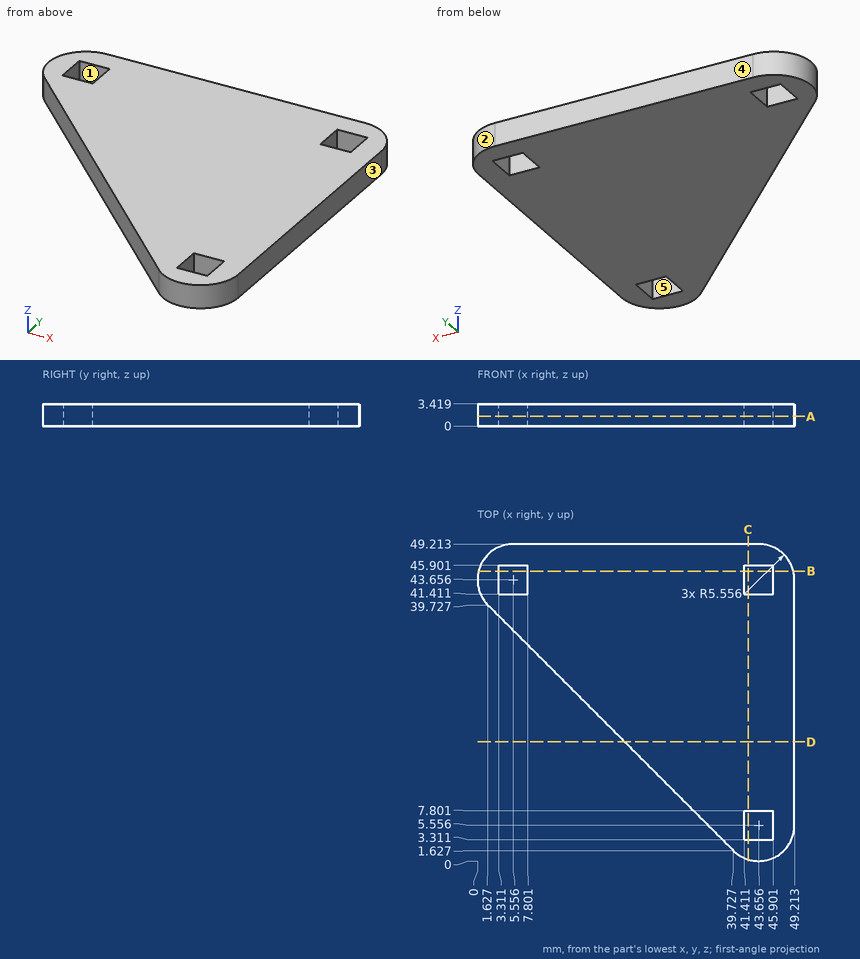
Source: three-view drawing plus pictorial views. Frame: mm from the lowest corner of the part. A direction names the side the tool comes from. Round coordinates to 2 decimals unless told otherwise and drop trailing zeros. Order: outer loops, then holes, each group sorted by start corner. A loop starts at its lowest first (then second) coordinate and runs counter-clockwise, first axis right, second up. Notation, with made-up numbers: (37.5, 24) -> (81.5, 24) arc R20 ccw to (81.5, 46) -> close; hole circle Ø9 at (67, 70). An arc over 180 degrees is marked (long way). Use CSV: the item, a comma, the result in double quotes. Start each with the question number.
1) Material intervals for line 1 along X through (y, z) = (44, 2.8); line 2 along X through (y, z) = (41.5, 2.4) (1 decimal), sorted ascending. Write a range as from..to.
2) Section D-D (y = 18.5). Return the cut outline in (x, z) (1 decimal).
3) Draft query along Y for the marked faces 1, 2 and 3. Return one class per face: +Y half, -Y half, draft (parallel to the pull), parting line (faces both ways), or undercut.
4) Section B-B (y = 45). Return the cut outline in (x, z) (1 decimal).
5) Set-up query: the marked faces 4 and 5. Return all of +Z, -Z, +X, -X, +Y, -Y with unobstructed straight access to the full face (end or side cutting, diameter ignored); none if empty.
6) Section C-C (x = 42). Return the cut outline in (y, z), and give its area (3 significant figures).
7) First-contact query: pin 1 Ø1.7 at (y, z) = (43, 1.5) entering from -X; pin 2 Ø1.5 at (x, z) = (12.5, 2.5) entering from -Y (1 decimal); pin 3 Ø1 at (y, z) = (4.5, 1.5) entering from -X (1 decimal). Flat tips, straight axial feed; report the tip coordinate or a pass-through.
8) Section A-A (z = 1.5). Return the cut outline in (x, y).
Returned:
1,line 1,"x = 0.01..3.31, 7.8..41.41, 45.9..49.2"
1,line 2,"x = 0.4..3.3, 7.8..41.4, 45.9..49.2"
2,outline,"(22.9, 0) -> (49.2, 0) -> (49.2, 3.4) -> (22.9, 3.4) -> close"
3,face 1,"undercut"
3,face 2,"+Y half"
3,face 3,"draft"
4,outline,"(0.2, 0) -> (3.3, 0) -> (3.3, 3.4) -> (0.2, 3.4) -> close; (7.8, 0) -> (41.4, 0) -> (41.4, 3.4) -> (7.8, 3.4) -> close; (45.9, 0) -> (49, 0) -> (49, 3.4) -> (45.9, 3.4) -> close"
5,face 4,"+Z, -Z, +X, -X, +Y"
5,face 5,"+Z, -Z"
6,outline,"(0.25, 0) -> (3.31, 0) -> (3.31, 3.42) -> (0.25, 3.42) -> close; (7.8, 0) -> (41.41, 0) -> (41.41, 3.42) -> (7.8, 3.42) -> close; (45.9, 0) -> (49.21, 0) -> (49.21, 3.42) -> (45.9, 3.42) -> close"
6,area,"137 mm²"
7,pin 1,"stops at x = 0"
7,pin 2,"stops at y = 28.1"
7,pin 3,"stops at x = 36.4"
8,outline,"(1.63, 39.73) -> (39.73, 1.63) arc R5.56 ccw to (49.21, 5.56) -> (49.21, 43.66) arc R5.56 ccw to (43.66, 49.21) -> (5.56, 49.21) arc R5.56 ccw to start; hole (3.31, 41.41) -> (7.8, 41.41) -> (7.8, 45.9) -> (3.31, 45.9) -> close; hole (41.41, 3.31) -> (45.9, 3.31) -> (45.9, 7.8) -> (41.41, 7.8) -> close; hole (41.41, 41.41) -> (45.9, 41.41) -> (45.9, 45.9) -> (41.41, 45.9) -> close"
